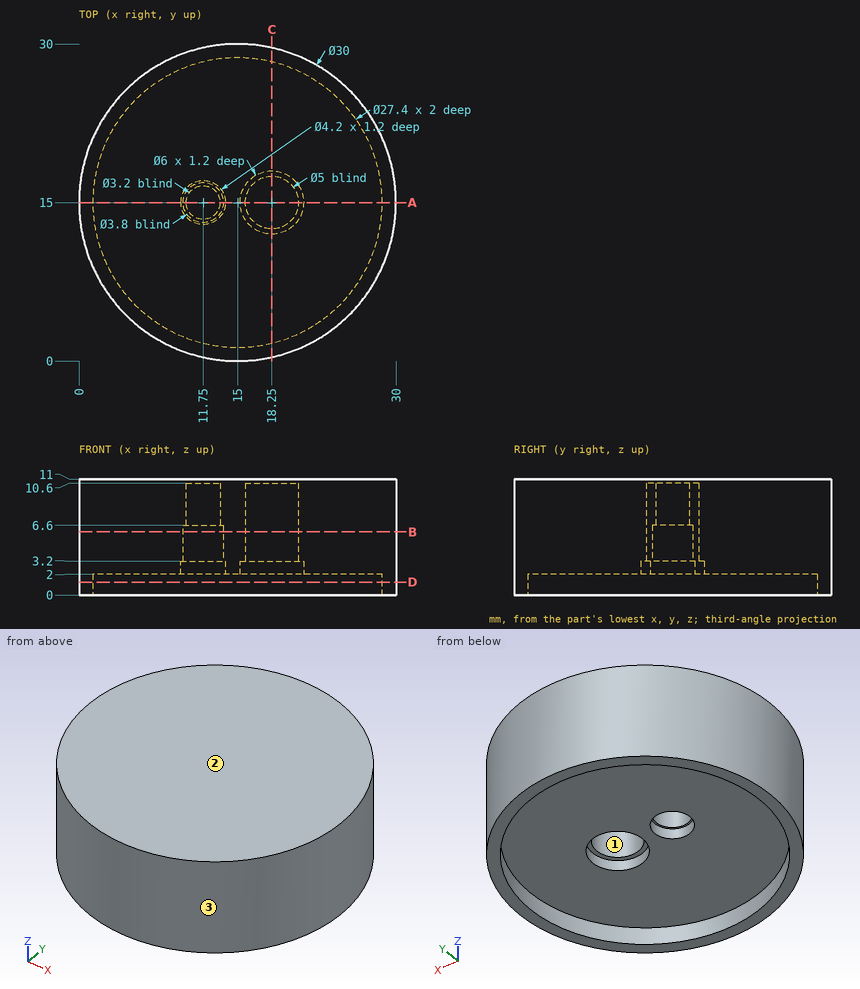
Design review of the part shown in the three views and the two pictorial views. Dimensions are in mm from the part's minimum x, y and z. Coordinates: 2 decimals unless noted, no trailing zeros. Write each loop counter-clockwise with the first axis right and the second up, starting at its lowest first coordinate (ties: lowest second). Pieces come first, ordered by that corner, then holes.
(1) Wall thickness on probe 1 along X at (y, z) = (14.5, 9.25); probe 2 along Z at (x, y) = (25, 20.75); probe 3 along X at (y, z) = (18.5, 1.75): over which ranges is each line inside the solid? List them lowest first.
(2) Add section C-C on x = 18.25. Give the boundary of the cut face in (y, z), then the cut area to 3 significant figures.
(3) For pin 1 Ø3 at (x, z) = (10, 5.5) entering from -Y; pin 2 Ø4 at (x, y) = (18, 16) entering from -Z; pin 3 Ø6 at (y, z) = (10, 9) entering from +X, all flat-tipped, find the tip position at first contact; note any pin that passes through.
(4) Add section A-A on y = 15. Give the boundary of the cut face in (x, z).
(5) Add section D-D on z = 1.25. Give the boundary of the cut face in (x, y), then the cut area to 3 significant figures.
(6) Add section B-B on z = 6. Give the boundary of the cut face in (x, y), then the cut area to 3 significant figures.
(7) The part is to be moulded in two halves that separate along Y. For the marked faces 1, 2 and 3, say which applies: +Y half, -Y half, draft (parallel to the pull), parting line (faces both ways), or undercut.
Answer sheet:
1. probe 1: x = 0.01 to 10.23, 13.27 to 15.8, 20.7 to 29.99
1. probe 2: z = 2 to 11
1. probe 3: x = 0.41 to 1.75, 28.25 to 29.59
2. outline: (0.36, 0) - (1.69, 0) - (1.69, 2) - (12, 2) - (12, 3.2) - (12.5, 3.2) - (12.5, 10.6) - (17.5, 10.6) - (17.5, 3.2) - (18, 3.2) - (18, 2) - (28.31, 2) - (28.31, 0) - (29.64, 0) - (29.64, 11) - (0.36, 11) - close
2. area: 225 mm2
3. pin 1: stops at y = 0.41
3. pin 2: stops at z = 2
3. pin 3: stops at x = 29.87
4. outline: (0, 0) - (1.3, 0) - (1.3, 2) - (9.65, 2) - (9.65, 3.2) - (9.85, 3.2) - (9.85, 6.6) - (10.15, 6.6) - (10.15, 10.6) - (13.35, 10.6) - (13.35, 6.6) - (13.65, 6.6) - (13.65, 3.2) - (13.85, 3.2) - (13.85, 2) - (15.25, 2) - (15.25, 3.2) - (15.75, 3.2) - (15.75, 10.6) - (20.75, 10.6) - (20.75, 3.2) - (21.25, 3.2) - (21.25, 2) - (28.7, 2) - (28.7, 0) - (30, 0) - (30, 11) - (0, 11) - close
5. outline: circle Ø30 at (15, 15); hole circle Ø27.4 at (15, 15)
5. area: 117 mm2
6. outline: circle Ø30 at (15, 15); hole circle Ø3.8 at (11.75, 15); hole circle Ø5 at (18.25, 15)
6. area: 676 mm2
7. face 1: undercut
7. face 2: draft
7. face 3: parting line
